Model file for the job. Use its own axes, mm. Face numbers are marked on the shaded views. Round coordinates to 2 decimals unless told otherwise and drop trailing zeros. Order: outer loops, then holes, each group sorted by start corner. A loop starts at its lowest first (then second) coordinate and runs counter-clockwise, first axis right, second up. Notation, with made-up numbers: (49, 49) -> (73, 49) arc R25 ccw to (73, 82) -> close; hole circle Ø3 at (-16, -34.5). An arc over 180 degrees is marked (long way). Use CSV: the item, a comma, the result in double quotes.
```python
from build123d import *

# Parameters (mm, degrees)
SKETCH1_R           = 1
BOSS_EXTRUDE1_DEPTH = 5
SKETCH2_W           = 5
SKETCH2_H           = 40
BOSS_EXTRUDE2_DEPTH = 80
SKETCH3_R           = 2.22
CUT_EXTRUDE3_DEPTH  = 80
SKETCH5_R           = 2.22
SKETCH5_R_2         = 1
BOSS_EXTRUDE3_DEPTH = 10
SKETCH6_R           = 3.5
SKETCH6_R_2         = 2.22
BOSS_EXTRUDE4_DEPTH = 5
SKETCH7_W           = 18.8
SKETCH7_H           = 4.557781783
CUT_EXTRUDE4_DEPTH  = 10
BOSS_EXTRUDE5_DEPTH = 5
SKETCH9_W           = 20
SKETCH9_H           = 6
CUT_EXTRUDE7_DEPTH  = 10
SKETCH10_W          = 5
SKETCH10_H          = 8
BOSS_EXTRUDE6_DEPTH = 10
SKETCH11_R          = 1
CUT_EXTRUDE9_DEPTH  = 8
SKETCH12_R          = 1
CUT_EXTRUDE10_DEPTH = 8


with BuildPart() as part:
    # Sketch1 → Boss-Extrude1 (new body)
    with BuildSketch(Plane(origin=(0, 0, 0), x_dir=(1, 0, 0), z_dir=(0, 1, 0))):
        with BuildLine():
            Line((5.319641756, -11.332905968), (15.319641756, -11.332905968))
            Line((15.319641756, -11.332905968), (15.319641756, 28.667094032))
            Line((15.319641756, 28.667094032), (5.319641756, 28.667094032))
            ThreePointArc((5.319641756, 28.667094032), (-1.751426056, 25.738161844), (-4.680358244, 18.667094032))
            Line((-4.680358244, 18.667094032), (-4.680358244, -1.332905968))
            ThreePointArc((-4.680358244, -1.332905968), (-1.751426056, -8.40397378), (5.319641756, -11.332905968))
        make_face()
        with Locations((5.319641756, 18.667094032)):
            Circle(SKETCH1_R, mode=Mode.SUBTRACT)
        with Locations((5.319641756, -1.332905968)):
            Circle(SKETCH1_R, mode=Mode.SUBTRACT)
    extrude(amount=BOSS_EXTRUDE1_DEPTH)

    # Sketch2 → Boss-Extrude2 (add)
    with BuildSketch(Plane(origin=(0, 5, 0), x_dir=(1, 0, 0), z_dir=(0, 1, 0))):
        with Locations((12.819641756, 8.667094032)):
            Rectangle(SKETCH2_W, SKETCH2_H)
    extrude(amount=BOSS_EXTRUDE2_DEPTH)

    # Sketch3 → Cut-Extrude3 (cut)
    with BuildSketch(Plane.ZY.offset(-10.319641756)):
        with BuildLine():
            ThreePointArc((0.732905968, 35.401978793), (1.440012749, 35.694872012), (1.732905968, 36.401978793))
            Line((1.732905968, 36.401978793), (1.732905968, 69.94419701))
            ThreePointArc((1.732905968, 69.94419701), (1.440012749, 70.651303792), (0.732905968, 70.94419701))
            Line((0.732905968, 70.94419701), (-18.067094032, 70.94419701))
            ThreePointArc((-18.067094032, 70.94419701), (-18.774200813, 70.651303792), (-19.067094032, 69.94419701))
            Line((-19.067094032, 69.94419701), (-19.067094032, 36.401978793))
            ThreePointArc((-19.067094032, 36.401978793), (-18.774200813, 35.694872012), (-18.067094032, 35.401978793))
            Line((-18.067094032, 35.401978793), (0.732905968, 35.401978793))
        make_face()
        with Locations((-13.167094032, 75.54419701)):
            Circle(SKETCH3_R)
        with Locations((-13.167094032, 25.24419701)):
            Circle(SKETCH3_R)
        with Locations((-4.167094032, 25.24419701)):
            Circle(SKETCH3_R)
        with Locations((-4.167094032, 75.54419701)):
            Circle(SKETCH3_R)
    extrude(amount=-CUT_EXTRUDE3_DEPTH, mode=Mode.SUBTRACT)

    # Sketch5 → Boss-Extrude3 (add)
    with BuildSketch(Plane(origin=(15.319641756, 0, 0), x_dir=(0, 0, -1), z_dir=(1, 0, 0))):
        with Locations((4.167094032, 25.24419701)):
            Circle(SKETCH5_R)
        with Locations((4.167094032, 25.24419701)):
            Circle(SKETCH5_R_2, mode=Mode.SUBTRACT)
        with Locations((13.167094032, 25.24419701)):
            Circle(SKETCH5_R)
        with Locations((13.167094032, 25.24419701)):
            Circle(SKETCH5_R_2, mode=Mode.SUBTRACT)
        with Locations((4.167094032, 75.54419701)):
            Circle(SKETCH5_R)
        with Locations((4.167094032, 75.54419701)):
            Circle(SKETCH5_R_2, mode=Mode.SUBTRACT)
        with Locations((13.167094032, 75.54419701)):
            Circle(SKETCH5_R)
        with Locations((13.167094032, 75.54419701)):
            Circle(SKETCH5_R_2, mode=Mode.SUBTRACT)
    extrude(amount=-BOSS_EXTRUDE3_DEPTH)

    # Sketch6 → Boss-Extrude4 (add)
    with BuildSketch(Plane.ZY.offset(-10.319641756)):
        with Locations((-4.167094032, 25.24419701)):
            Circle(SKETCH6_R)
        with Locations((-4.167094032, 25.24419701)):
            Circle(SKETCH6_R_2, mode=Mode.SUBTRACT)
        with Locations((-13.167094032, 25.24419701)):
            Circle(SKETCH6_R)
        with Locations((-13.167094032, 25.24419701)):
            Circle(SKETCH6_R_2, mode=Mode.SUBTRACT)
        with Locations((-4.167094032, 75.54419701)):
            Circle(SKETCH6_R)
        with Locations((-4.167094032, 75.54419701)):
            Circle(SKETCH6_R_2, mode=Mode.SUBTRACT)
        with Locations((-13.167094032, 75.54419701)):
            Circle(SKETCH6_R)
        with Locations((-13.167094032, 75.54419701)):
            Circle(SKETCH6_R_2, mode=Mode.SUBTRACT)
    extrude(amount=BOSS_EXTRUDE4_DEPTH)

    # Sketch7 → Cut-Extrude4 (cut)
    with BuildSketch(Plane.ZY.offset(-10.319641756)):
        with BuildLine():
            ThreePointArc((1.732905968, 36.401978793), (1.627333159, 35.954765198), (1.332905968, 35.601978793))
            Line((1.332905968, 35.601978793), (1.332905968, 30.84419701))
            ThreePointArc((1.332905968, 30.84419701), (1.157170037, 30.419932942), (0.732905968, 30.24419701))
            Line((0.732905968, 30.24419701), (-18.067094032, 30.24419701))
            ThreePointArc((-18.067094032, 30.24419701), (-18.491358101, 30.419932942), (-18.667094032, 30.84419701))
            Line((-18.667094032, 30.84419701), (-18.667094032, 35.601978793))
            ThreePointArc((-18.667094032, 35.601978793), (-18.961521223, 35.954765198), (-19.067094032, 36.401978793))
            Line((-19.067094032, 36.401978793), (-19.067094032, 30.84419701))
            ThreePointArc((-19.067094032, 30.84419701), (-18.774200813, 30.137090229), (-18.067094032, 29.84419701))
            Line((-18.067094032, 29.84419701), (0.732905968, 29.84419701))
            ThreePointArc((0.732905968, 29.84419701), (1.440012749, 30.137090229), (1.732905968, 30.84419701))
            Line((1.732905968, 30.84419701), (1.732905968, 36.401978793))
        make_face()
        with BuildLine():
            Line((1.332905968, 30.84419701), (1.332905968, 35.601978793))
            ThreePointArc((1.332905968, 35.601978793), (1.049133734, 35.453295495), (0.732905968, 35.401978793))
            Line((0.732905968, 35.401978793), (0.732905968, 30.84419701))
            Line((0.732905968, 30.84419701), (-18.067094032, 30.84419701))
            Line((-18.067094032, 30.84419701), (-18.067094032, 35.401978793))
            ThreePointArc((-18.067094032, 35.401978793), (-18.383321798, 35.453295495), (-18.667094032, 35.601978793))
            Line((-18.667094032, 35.601978793), (-18.667094032, 30.84419701))
            ThreePointArc((-18.667094032, 30.84419701), (-18.491358101, 30.419932942), (-18.067094032, 30.24419701))
            Line((-18.067094032, 30.24419701), (0.732905968, 30.24419701))
            ThreePointArc((0.732905968, 30.24419701), (1.157170037, 30.419932942), (1.332905968, 30.84419701))
        make_face()
        with Locations((-8.667094032, 33.123087901)):
            Rectangle(SKETCH7_W, SKETCH7_H)
    extrude(amount=-CUT_EXTRUDE4_DEPTH, mode=Mode.SUBTRACT)

    # Sketch8 → Boss-Extrude5 (add, through all)
    with BuildSketch(Plane.ZY.offset(-10.319641756)):
        Polygon((-28.667094032, 89.50779106), (-28.667094032, 85), (-16.300533883, 85), (-16.300533883, 94.015582119), align=None)
        Polygon((-1.033654181, 94.015582119), (-1.033654181, 85), (11.332905968, 85), (11.332905968, 89.50779106), align=None)
    extrude(amount=-BOSS_EXTRUDE5_DEPTH)

    # Sketch9 → Cut-Extrude7 (cut)
    with BuildSketch(Plane.ZY.offset(-10.319641756)):
        with Locations((-8.667094032, 13)):
            Rectangle(SKETCH9_W, SKETCH9_H)
    extrude(amount=-CUT_EXTRUDE7_DEPTH, mode=Mode.SUBTRACT)

    # Sketch10 → Boss-Extrude6 (add)
    with BuildSketch(Plane.ZY.offset(-10.319641756)):
        with Locations((-25.767094032, 17.566871705)):
            Rectangle(SKETCH10_W, SKETCH10_H)
        with Locations((8.432905968, 17.566871705)):
            Rectangle(SKETCH10_W, SKETCH10_H)
        with Locations((8.432905968, 75.6)):
            Rectangle(SKETCH10_W, SKETCH10_H)
        with Locations((-25.767094032, 75.6)):
            Rectangle(SKETCH10_W, SKETCH10_H)
    extrude(amount=BOSS_EXTRUDE6_DEPTH)

    # Sketch11 → Cut-Extrude9 (cut)
    with BuildSketch(Plane.XY.offset(10.932905968)):
        with Locations((5.319641756, 17.566871705)):
            Circle(SKETCH11_R)
        with Locations((5.319641756, 75.6)):
            Circle(SKETCH11_R)
    extrude(amount=-CUT_EXTRUDE9_DEPTH, mode=Mode.SUBTRACT)

    # Sketch12 → Cut-Extrude10 (cut)
    with BuildSketch(Plane(origin=(0, 0, -28.267094032), x_dir=(-1, 0, 0), z_dir=(0, 0, -1))):
        with Locations((-5.319641756, 75.6)):
            Circle(SKETCH12_R)
        with Locations((-5.319641756, 17.566871705)):
            Circle(SKETCH12_R)
    extrude(amount=-CUT_EXTRUDE10_DEPTH, mode=Mode.SUBTRACT)


solid = part.part
```
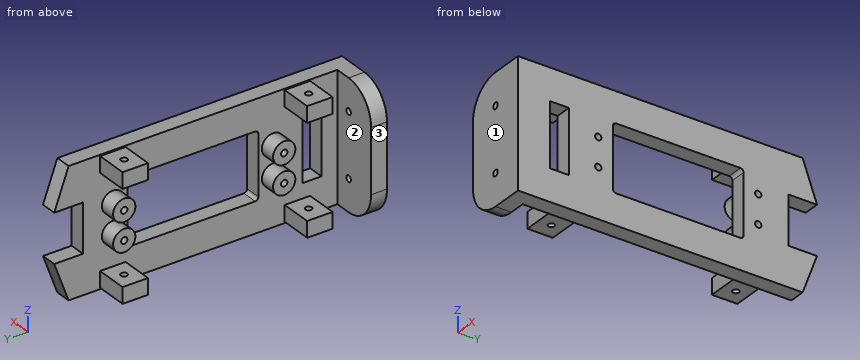
Q1. Probe line 1 along Y through (x, z) = (14, -15.5); line 2 along Y through (x, z) = (6.75, 9); line 3 along Z through (x, y) = (13.5, 46.5). List the from-to ranges inside material, lowest first.
From the geometry:
line 1,"y = 0 to 10, 16 to 29.84, 70.94 to 85"
line 2,"y = 0 to 5, 13.57 to 21.57, 71.6 to 79.6"
line 3,"z = -28.67 to -19.07, 1.73 to 11.33"
Q2. Cut at D-D (z = -15). Give the cut face in (x, y).
From the geometry:
outline,"(-4.68, 0) -> (15.32, 0) -> (15.32, 10) -> (10.32, 10) -> (10.32, 5) -> (-4.68, 5) -> close; (5.32, 22.26) -> (10.32, 22.26) -> (10.32, 16) -> (15.32, 16) -> (15.32, 29.84) -> (10.32, 29.84) -> (10.32, 28.23) -> (5.32, 28.23) -> close; (5.32, 72.56) -> (10.32, 72.56) -> (10.32, 70.94) -> (15.32, 70.94) -> (15.32, 85) -> (10.32, 85) -> (10.32, 78.53) -> (5.32, 78.53) -> close"
Q3. Cut at C-C (y = 20.5). Give the cut face in (x, z).
From the geometry:
outline,"(0.32, -28.27) -> (10.32, -28.27) -> (10.32, -28.67) -> (15.32, -28.67) -> (15.32, 11.33) -> (10.32, 11.33) -> (10.32, 10.93) -> (0.32, 10.93) -> (0.32, 5.93) -> (10.32, 5.93) -> (10.32, -23.27) -> (0.32, -23.27) -> close"
Q4. Mould opens along Y. For the marked faces 1, 2 and 3 say: +Y half, -Y half, draft (parallel to the pull), parting line (faces both ways), or undercut.
From the geometry:
face 1,"-Y half"
face 2,"undercut"
face 3,"draft"
Q5. Cut at B-B (x = 7.5). State how many separate pieces and enclosed holes the cut face has, plus the area to 3 significant figures.
From the geometry:
separate pieces,"9"
enclosed holes,"4"
area,"501 mm²"
Q6. Cut at A-A (y = 56). Give the cut face in (x, z), plus the area to 3 significant figures.
From the geometry:
outline,"(10.32, -28.67) -> (15.32, -28.67) -> (15.32, -19.07) -> (10.32, -19.07) -> close; (10.32, 1.73) -> (15.32, 1.73) -> (15.32, 11.33) -> (10.32, 11.33) -> close"
area,"96.0 mm²"
Q7. Pin check, flat tips, straight feed: pin 1 (1.2 mm diameter, centred on x = 5.32, y = 75.6, fed in from +Z); pin 2 (4 mm diameter, centred on x = 13, z = -11.5, fed in from +Y); pin 3 (1.8 mm diameter, centred on x = 5.32, y = 17.57, fed in from +Z); pin 4 (20 mm diameter, centred on y = 61.5, z = -2, fed in from -X). Stop position of each tip, or through.
From the geometry:
pin 1,"stops at z = -0.67"
pin 2,"stops at y = 85"
pin 3,"passes through"
pin 4,"stops at x = 10.32"
